Autodesk Inventor part; units mm, degrees
ref_plane "YZ Plane" through (0, 0, 0) normal (1, 0, 0) x (0, 1, 0)
ref_plane "XZ Plane" through (0, 0, 0) normal (0, 1, 0) x (-1, 0, 0)
ref_plane "XY Plane" through (0, 0, 0) normal (0, 0, 1) x (1, 0, 0)
sketch "Sketch1" plane through (0, 0, 0) normal (0, 0, 1) x (1, 0, 0)
  line L0 (0, 0) -> (5, 0)
  line L1 (5, 0) -> (-5, 0)
  circle A0 centre (-5, 0) radius 1.75
  circle A1 centre (5, 0) radius 1.75
  line L2 (0, 0) -> (0, -5)
  line L3 (0, -5) -> (11, -5)
  line L4 (11, -5) -> (11, 5)
  line L5 (0, -5) -> (-10, -5)
  line L6 (-10, -5) -> (-10, 5)
  line L7 (11, 5) -> (7.2436, 15.3207)
  line L8 (11, 5) -> (21.9831, 5) construction
  line L9 (6.2581, 32.5632) -> (10.8155, 51.6081)
  line L10 (9.9731, 53.7422) -> (8.756, 54.5465)
  line L11 (1.1367, 51.5387) -> (-10, 5)
  arc A2 (6.2581, 32.5632) -> (7.2436, 15.3207) centre (35.4343, 25.5813) ccw
  arc A3 (10.8155, 51.6081) -> (9.9731, 53.7422) centre (8.8705, 52.0736) ccw
  arc A4 (8.756, 54.5465) -> (1.1367, 51.5387) centre (5.9994, 50.375) ccw
  point P0 (4.1596, 23.7939)
  point P1 (11.1415, 52.9701)
  point P2 (2.7985, 58.4833)
  dimension "d0" = 5
  dimension "d1" = 10
  dimension "d2" = 3.5
  dimension "d3" = 3.5
  dimension "d4" = 5
  dimension "d5" = 11
  dimension "d6" = 10
  dimension "d7" = 10
  dimension "d8" = 10
  dimension "d9" = 20
  dimension "d10" = 110
  dimension "d11" = 30
  dimension "d12" = 10
  dimension "d13" = 110
  dimension "d14" = 30
  dimension "d15" = 2
  dimension "d16" = 5
extrude "Extrusion1" add sketch "Sketch1" along normal blind 5
properties part number "gripper"
CAD build for the part. Positions are in the model's coordinates, mm. A direction names the side the tool comes from. Coordinates: 2 decimals unless noted, no trailing zeros. Loops run counter-clockwise (first coordinate to the right, second up) from the corner with the lowest first, then second, coordinate; pieces in that order, holes last. Notation, with made-up numbers: (-17, 16) -> (7, 16) arc R9 cw to (7, 25) -> close; hole circle Ø1 at (-7, -36.75). An arc over 180 degrees is marked (long way). One line per item, written item: value.
1. Pull direction Y, two halves, no side cores. Call faces 1 (the face through (-6.75, -0.08, 2.46)), 2 (the face through (11, 0, 2)), 3 (the face through (10.724, 52.824, 2.465)), 4 (the face through (4.1, 55, 2.5)): pulls with the +Y half, pulls with the -Y half, needs draft (parallel to the pull), parting line crosses it, or undercut.
Answers:
face 1: undercut
face 2: needs draft
face 3: undercut
face 4: pulls with the +Y half
2. Slice it at B-B on z = 3.5. Write the cut outline in (x, y).
Answers:
outline: (-10, -5) -> (11, -5) -> (11, 5) -> (7.24, 15.32) arc R30 cw to (6.26, 32.56) -> (10.82, 51.61) arc R2 ccw to (9.97, 53.74) -> (8.76, 54.55) arc R5 ccw to (1.14, 51.54) -> (-10, 5) -> close; hole circle Ø3.5 at (-5, 0); hole circle Ø3.5 at (5, 0)
3. Flat gauge pin, fed straight in: P1, Ø3, axis at x = 1, z = 1, coming from the +Y side. Where does the tip first touch, or does it go through?
Answers:
P1: stops at y = 53.95
4. Slice it at C-C on x = -5. Write the cut outline in (y, z).
Answers:
outline: (-5, 0) -> (-1.75, 0) -> (-1.75, 5) -> (-5, 5) -> close; (1.75, 0) -> (25.89, 0) -> (25.89, 5) -> (1.75, 5) -> close
5. Which spindle directions (+Z, -Z, +X, -X, +Y, -Y) get a long thin tool onto all of the face, cutting with end or side? Do faces 5 (the face through (8.505, 41.952, 2.465)), 6 (the face through (9.37, 54.14, 2.46)). Say none if no direction does.
Answers:
face 5: +Z, -Z, +X
face 6: +Z, -Z, +X, +Y
6. Slice it at D-D on y = 20.5. Write the cut outline in (x, z), and give its area (3 significant figures).
Answers:
outline: (-6.29, 0) -> (5.87, 0) -> (5.87, 5) -> (-6.29, 5) -> close
area: 60.8 mm^2
7. Slice it at A-A on y = 0. Write the cut outline in (x, z).
Answers:
outline: (-10, 0) -> (-6.75, 0) -> (-6.75, 5) -> (-10, 5) -> close; (-3.25, 0) -> (3.25, 0) -> (3.25, 5) -> (-3.25, 5) -> close; (6.75, 0) -> (11, 0) -> (11, 5) -> (6.75, 5) -> close
8. Drill centre lines: line 1 (Y direction, x = 5, z = 3.75); line 2 (X direction, y = 27, z = 0.8); line 3 (X direction, y = 46.5, z = 3.8). Where is each one in solid material? Low to high. Write a range as [from, to].
Answers:
line 1: y = [-5, -1.75], [1.75, 55.27]
line 2: x = [-4.74, 5.47]
line 3: x = [-0.07, 9.59]
